from build123d import *

# Parameters (mm, degrees)
F1_DEPTH = 63.5
F3_D     = 10.922


with BuildPart() as f1:
    # F0 (on Top) → F1 (new body)
    with BuildSketch(Plane.XY):
        with BuildLine():
            ThreePointArc((-10.3378, 12.7), (-12.008128, 12.008128), (-12.7, 10.3378))
            Line((-12.7, 10.3378), (-12.7, -10.3378))
            ThreePointArc((-12.7, -10.3378), (-12.008128, -12.008128), (-10.3378, -12.7))
            Line((-10.3378, -12.7), (10.3378, -12.7))
            ThreePointArc((10.3378, -12.7), (12.008128, -12.008128), (12.7, -10.3378))
            Line((12.7, -10.3378), (12.7, 10.3378))
            ThreePointArc((12.7, 10.3378), (12.008128, 12.008128), (10.3378, 12.7))
            Line((10.3378, 12.7), (-10.3378, 12.7))
        make_face()
        with BuildLine():
            Line((-8.8138, 10.3378), (8.8138, 10.3378))
            ThreePointArc((8.8138, 10.3378), (9.891431, 9.891431), (10.3378, 8.8138))
            Line((10.3378, 8.8138), (10.3378, -8.8138))
            ThreePointArc((10.3378, -8.8138), (9.891431, -9.891431), (8.8138, -10.3378))
            Line((8.8138, -10.3378), (-8.8138, -10.3378))
            ThreePointArc((-8.8138, -10.3378), (-9.891431, -9.891431), (-10.3378, -8.8138))
            Line((-10.3378, -8.8138), (-10.3378, 8.8138))
            ThreePointArc((-10.3378, 8.8138), (-9.891431, 9.891431), (-8.8138, 10.3378))
        make_face(mode=Mode.SUBTRACT)
    extrude(amount=F1_DEPTH)

    # F3 (through all)
    with Locations(Plane.XZ.offset(12.7)):
        with Locations((0, 31.75)):
            Hole(F3_D / 2)


solid = f1.part
Could you check a few things on this model? Use its own coordinates, in mm. A direction names the side the tool comes from. Give positions to 0.01 mm unless a question says otherwise; leave off trailing zeros. Order: outer loops, then holes, each group sorted by start corner. A loop starts at its lowest first (then second) coordinate and runs counter-clockwise, first axis right, second up. Notation, with made-up numbers: (9.25, 69.25) - (47.25, 69.25) arc R21 cw to (47.25, 102.25) - close; hole circle Ø8 at (-27, 31.5). An arc over 180 degrees is marked (long way). Return JSON: item names as keys, results as strings. Group by question number.
Q1. Thinking about a two-plate mould opening in Z: for faces 3 (the face through (9.88, 9.9, 31.31)), 4 (the face through (1.18, -11.5, 26.42)), 5 (the face through (11, 0, 63.5)), 6 (the face through (1.18, 11.54, 26.42)), which applies, pulls with the +Z half, pulls with the -Z half, needs draft (parallel to the pull), parting line crosses it, or undercut?
Q2. Suppose I cut it at B-B, the plane z = 31.75. Please give me the cut outline in (x, y), and give its area (3 significant figures).
Q3. Please list where these lines run through material, in increasing order: line 1 along X through (y, z) = (-6.25, 61.5); line 2 along Z through (x, y) = (0, 12). Write a range as [from, to].
Q4. Suppose I cut it at D-D, the plane z = 60. Please give me the cut outline in (x, y).
Q5. Will this pin go through, and if not, where does the flat tip stop? pin 1 Ø9 at (x, z) = (-3, 34.5) entering from +Y.
Q6. Which directions (+Z, -Z, +X, -X, +Y, -Y) give clear straight access to the entire face, cutting with the end or side of a thin tool? Please do faces 1 (the face through (12.7, 0, 31)), 2 (the face through (-6, -10.338, 31)).
Q7. Suppose I cut it at A-A, the plane x = 0. Please give me the cut outline in (y, z), and give its area (3 significant figures).
Q8. Suppose I cut it at C-C, the plane x = 7. Please give me the cut outline in (y, z).
Resolved:
{
 "1": {"face 3": "needs draft", "face 4": "undercut", "face 5": "pulls with the +Z half", "face 6": "undercut"},
 "2": {"outline": "(-12.7, -10.34) arc R2.36 ccw to (-10.34, -12.7) - (-5.46, -12.7) - (-5.46, -10.34) - (-8.81, -10.34) arc R1.52 cw to (-10.34, -8.81) - (-10.34, 8.81) arc R1.52 cw to (-8.81, 10.34) - (-5.46, 10.34) - (-5.46, 12.7) - (-10.34, 12.7) arc R2.36 ccw to (-12.7, 10.34) - close; (5.46, -12.7) - (10.34, -12.7) arc R2.36 ccw to (12.7, -10.34) - (12.7, 10.34) arc R2.36 ccw to (10.34, 12.7) - (5.46, 12.7) - (5.46, 10.34) - (8.81, 10.34) arc R1.52 cw to (10.34, 8.81) - (10.34, -8.81) arc R1.52 cw to (8.81, -10.34) - (5.46, -10.34) - close", "area": "163 mm2"},
 "3": {"line 1": "x = [-12.7, -10.34], [10.34, 12.7]", "line 2": "z = [0, 26.29], [37.21, 63.5]"},
 "4": {"outline": "(-12.7, -10.34) arc R2.36 ccw to (-10.34, -12.7) - (10.34, -12.7) arc R2.36 ccw to (12.7, -10.34) - (12.7, 10.34) arc R2.36 ccw to (10.34, 12.7) - (-10.34, 12.7) arc R2.36 ccw to (-12.7, 10.34) - close; hole (-10.34, -8.81) arc R1.52 ccw to (-8.81, -10.34) - (8.81, -10.34) arc R1.52 ccw to (10.34, -8.81) - (10.34, 8.81) arc R1.52 ccw to (8.81, 10.34) - (-8.81, 10.34) arc R1.52 ccw to (-10.34, 8.81) - close"},
 "5": {"pin 1": "stops at y = 12.7"},
 "6": {"face 1": "+Z, -Z, +X, +Y, -Y", "face 2": "+Z, -Z"},
 "7": {"outline": "(-12.7, 0) - (-10.34, 0) - (-10.34, 26.29) - (-12.7, 26.29) - close; (-12.7, 37.21) - (-10.34, 37.21) - (-10.34, 63.5) - (-12.7, 63.5) - close; (10.34, 0) - (12.7, 0) - (12.7, 26.29) - (10.34, 26.29) - close; (10.34, 37.21) - (12.7, 37.21) - (12.7, 63.5) - (10.34, 63.5) - close", "area": "248 mm2"},
 "8": {"outline": "(-12.7, 0) - (-10.34, 0) - (-10.34, 63.5) - (-12.7, 63.5) - close; (10.34, 0) - (12.7, 0) - (12.7, 63.5) - (10.34, 63.5) - close"}
}
